```python
from build123d import *

# Parameters (mm, degrees)
BOSS_EXTRUDE1_DEPTH = 5.08


with BuildPart() as part:
    # Sketch1 → Boss-Extrude1 (new body)
    with BuildSketch(Plane.XY):
        with BuildLine():
            Line((0.629745632, 0.007769029), (-31.749999049, 0.007769029))
            Line((-31.749999049, 0.007769029), (-31.749999049, -25.519230971))
            Line((-31.749999049, -25.519230971), (-24.897254295, -25.519230971))
            ThreePointArc((-24.897254295, -25.519230971), (-17.420569124, -7.468916193), (0.629745632, 0.007769029))
        make_face()
        with BuildLine():
            Line((31.749999049, 0.007769029), (0.629745632, 0.007769029))
            ThreePointArc((0.629745632, 0.007769029), (18.680060482, -7.468916142), (26.156745705, -25.519230971))
            Line((26.156745705, -25.519230971), (31.749999049, -25.519230971))
            Line((31.749999049, -25.519230971), (31.749999049, 0.007769029))
        make_face()
        with BuildLine():
            ThreePointArc((-31.749999049, 0.007769029), (0, 31.75), (31.749999049, 0.007769029))
            Line((31.749999049, 0.007769029), (-31.749999049, 0.007769029))
        make_face()
    extrude(amount=-BOSS_EXTRUDE1_DEPTH)


solid = part.part
```
Verification items for the finished model (mm, model axes). Coordinates: 2 decimals unless noted, no trailing zeros. Loops run counter-clockwise (first coordinate to the right, second up) from the corner with the lowest first, then second, coordinate; pieces in that order, holes last. Notation, with made-up numbers: (8.5, -7.5) - (32.5, -7.5) arc R7 cw to (32.5, 1.5) - close; hole circle Ø2 at (32.25, 30.5). An arc over 180 degrees is marked (long way). Answer as a JSON object with one key per item and string values.
(1) Go/stop test with a flat-tipped pin: pin 1 Ø1.5 at (x, z) = (13.5, -3.5) entering from +Y. Record where the tip stops, or that it passes through.
Response:
{"pin 1": "stops at y = 29.08"}
(2) Cross-section at B-B, the plane y = -6. Record the boundary of the cut face in (x, z).
Response:
{"outline": "(-31.75, -5.08) - (-15.82, -5.08) - (-15.82, 0) - (-31.75, 0) - close; (17.08, -5.08) - (31.75, -5.08) - (31.75, 0) - (17.08, 0) - close"}
(3) Cross-section at C-C, the plane x = 23. Record the boundary of the cut face in (y, z).
Response:
{"outline": "(-13.22, -5.08) - (21.89, -5.08) - (21.89, 0) - (-13.22, 0) - close"}
(4) Scan lines: line 1 along X through (y, z) = (-8, -3.35); line 2 along X through (y, z) = (-2.5, -4.7); line 3 along X through (y, z) = (3.5, -3.6). Record each from-to range of solid material in increasing order.
Response:
{"line 1": "x = -31.75 to -17.94, 19.2 to 31.75", "line 2": "x = -31.75 to -10.4, 11.66 to 31.75", "line 3": "x = -31.56 to 31.56"}
(5) Cross-section at A-A, the plane z = -1.05. Record the boundary of the cut face in (x, y), then the cut area to 3 significant figures.
Response:
{"outline": "(-31.75, -25.52) - (-24.9, -25.52) arc R25.53 cw to (26.16, -25.52) - (31.75, -25.52) - (31.75, 0.01) arc R31.75 ccw to (-31.75, 0.01) - close", "area": "2,180 mm²"}
(6) Cross-section at D-D, the plane y = -19. Record the boundary of the cut face in (x, z).
Response:
{"outline": "(-31.75, -5.08) - (-24.05, -5.08) - (-24.05, 0) - (-31.75, 0) - close; (25.31, -5.08) - (31.75, -5.08) - (31.75, 0) - (25.31, 0) - close"}
